Geometry check sheet. Reference: the model listing, model coordinates, mm. Face numbers are marked on the shaded views. Round coordinates to 2 decimals unless told otherwise and drop trailing zeros. Loops run counter-clockwise (first coordinate to the right, second up) from the corner with the lowest first, then second, coordinate; pieces in that order, holes last. Notation, with made-up numbers: (-33.5, 29) - (-13.5, 29) arc R16 ccw to (-13.5, 43) - close; hole circle Ø3 at (63.5, 43.25). An arc over 180 degrees is marked (long way). Answer as CSV lines item,"result". Start each with the question number.
1) Cross-section at C-C on x = -92.5. Record the boundary of the cut face in (y, z).
2) Cross-section at B-B on z = -218.5. Record the boundary of the cut face in (x, y).
3) Cross-section at A-A on y = 7. Record the boundary of the cut face in (x, z).
4) Draft check along X on the marked faces 1 and 2. Enter one of: released by +X, released by -X, zero draft, split by the parting line, or undercut.
5) Thickness scan on line 1 along X through (y, z) = (5.25, 234); line 2 along X through (y, z) = (9.25, -265); line 3 along Y through (x, z) = (-187.5, -121.5). Record the ranges inside material, lowest first.
6) Depth check by flat-ended pin: P1, Ø4.5, axis at x = -352, z = -127, coming from the -Y side; P2, Ø8, axis at x = -6, z = 194, coming from the +Y side. Enter the tip coordinate at first touch or a pass-through.
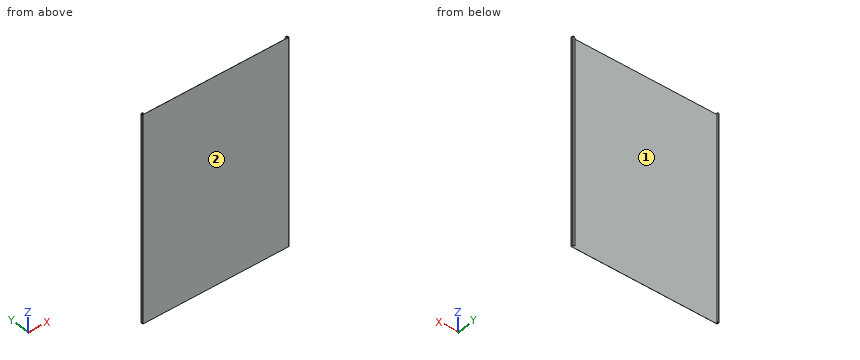
Autodesk Inventor part; units mm, degrees
ref_plane "YZ Plane" through (0, 0, 0) normal (1, 0, 0) x (0, 1, 0)
ref_plane "XZ Plane" through (0, 0, 0) normal (0, 1, 0) x (-1, 0, 0)
ref_plane "XY Plane" through (0, 0, 0) normal (0, 0, 1) x (1, 0, 0)
sketch "Sketch6" plane through (0, 0, 0) normal (0, 1, 0) x (-1, 0, 0)
  line L0 (356.7, -490) -> (-356.7, -490)
  line L1 (-356.7, -490) -> (-356.7, 490)
  line L2 (-356.7, 490) -> (356.7, 490)
  line L3 (356.7, 490) -> (356.7, -490)
  line L4 (356.7, -490) -> (-356.7, 490) construction
  line L5 (-356.7, -490) -> (356.7, 490) construction
  point P0 (0, 0)
  dimension "d52" = 713.4
  dimension "d53" = 980
extrude "Plate2" add sketch "Sketch6" along normal blind 0.5
sketch "Sketch11" plane through (-356.2, 0, 490) normal (-1, 0, 0) x (0, -1, 0)
  line L0 (0, -980) -> (0, 0)
  line L1 (0, 0) -> (-10, 0)
  line L2 (-10, 0) -> (-10, -980)
  line L3 (-10, -980) -> (0, -980)
edge flange "Flange2" height 10 angle 90 thickness 0.5 bend radius 0.5 thickness toward (-1, 0, 0) relief tear relief width 0.5 relief depth 0.25 edges at (-356.7, 0.5, 0) wall of the first edge with corners at (-356.2, 0, -490) (-356.2, 0, 490) (-356.2, 10, 490) (-356.2, 10, -490)
bend "Bend3"
corner "Corner3"
sketch "Sketch12" plane through (-356.7, 9.5, 490) normal (0, 1, 0) x (-1, 0, 0)
  line L0 (0, -980) -> (0, 0)
  line L1 (0, 0) -> (-10, 0)
  line L2 (-10, 0) -> (-10, -980)
  line L3 (-10, -980) -> (0, -980)
edge flange "Flange3" height 10 angle 90 thickness 0.5 bend radius 0.5 thickness toward (0, 1, 0) relief tear relief width 0.5 relief depth 0.25 edges at (-356.2, 10, 0) wall of the first edge with corners at (-356.7, 9.5, -490) (-356.7, 9.5, 490) (-346.7, 9.5, 490) (-346.7, 9.5, -490)
bend "Bend4"
corner "Corner4"
sketch "Sketch13" plane through (356.2, 0, -490) normal (1, 0, 0) x (0, 1, 0)
  line L0 (0, 980) -> (0, 0)
  line L1 (0, 0) -> (10, 0)
  line L2 (10, 0) -> (10, 980)
  line L3 (10, 980) -> (0, 980)
edge flange "Flange4" height 10 angle 90 thickness 0.5 bend radius 0.5 thickness toward (1, 0, 0) relief tear relief width 0.5 relief depth 0.25 edges at (356.7, 0.5, 0) wall of the first edge with corners at (356.2, 0, 490) (356.2, 0, -490) (356.2, 10, -490) (356.2, 10, 490)
bend "Bend5"
corner "Corner5"
sketch "Sketch14" plane through (356.7, 9.5, -490) normal (0, 1, 0) x (-1, 0, 0)
  line L0 (0, 980) -> (0, 0)
  line L1 (0, 0) -> (10, 0)
  line L2 (10, 0) -> (10, 980)
  line L3 (10, 980) -> (0, 980)
edge flange "Flange5" height 10 angle 90 thickness 0.5 bend radius 0.5 thickness toward (0, 1, 0) relief tear relief width 0.5 relief depth 0.25 edges at (356.2, 10, 0) wall of the first edge with corners at (356.7, 9.5, 490) (356.7, 9.5, -490) (346.7, 9.5, -490) (346.7, 9.5, 490)
bend "Bend6"
corner "Corner6"
fillet "Corner Round1" radius 4 4 edges at (346.7, 9.75, -490) (346.7, 9.75, 490) (-346.7, 9.75, -490) (-346.7, 9.75, 490)
equation "\"d52\" = ЖАБРЫ_базовая_ширина - 2 * ЖАБРЫ_шаг_листов"
equation "\"d53\" = ЖАБРЫ_базовая_длина_кор_лист"
equation "\"d54\" = Thickness"
equation "\"d84\" = BendReliefWidth"
equation "\"d85\" = BendReliefDepth"
equation "\"d86\" = MinimumRemnant"
equation "\"d87\" = TransitionRadius"
equation "\"d90\" = BendRadius"
equation "\"d91\" = CornerReliefSize"
equation "\"d92\" = GapSize"
equation "\"d93\" = JacobiRadiusSize"
equation "\"d94\" = BendReliefWidth"
equation "\"d95\" = BendReliefDepth"
equation "\"d96\" = MinimumRemnant"
equation "\"d97\" = TransitionRadius"
equation "\"d100\" = BendRadius"
equation "\"d101\" = CornerReliefSize"
equation "\"d102\" = GapSize"
equation "\"d103\" = JacobiRadiusSize"
equation "\"d104\" = BendReliefWidth"
equation "\"d105\" = BendReliefDepth"
equation "\"d106\" = MinimumRemnant"
equation "\"d107\" = TransitionRadius"
equation "\"d110\" = BendRadius"
equation "\"d111\" = CornerReliefSize"
equation "\"d112\" = GapSize"
equation "\"d113\" = JacobiRadiusSize"
equation "\"d114\" = BendReliefWidth"
equation "\"d115\" = BendReliefDepth"
equation "\"d116\" = MinimumRemnant"
equation "\"d117\" = TransitionRadius"
equation "\"d120\" = BendRadius"
equation "\"d121\" = CornerReliefSize"
equation "\"d122\" = GapSize"
equation "\"d123\" = JacobiRadiusSize"
equation "\"BendRadius\" = Thickness"
equation "\"BendReliefWidth\" = Thickness"
equation "\"BendReliefDepth\" = 0.5 * Thickness"
equation "\"CornerReliefSize\" = 4 * Thickness"
equation "\"MinimumRemnant\" = 2 * Thickness"
equation "\"TransitionRadius\" = BendRadius"
equation "\"JacobiRadiusSize\" = BendRadius"
equation "\"GapSize\" = Thickness"
properties part number "MSC 806 SHEET GILLS" material "Stainless Steel"
Answer block:
1,outline,"(0, -490) - (0.5, -490) - (0.5, 490) - (0, 490) - close"
2,outline,"(-356.7, 1) arc R1 ccw to (-355.7, 0) - (355.7, 0) arc R1 ccw to (356.7, 1) - (356.7, 9) arc R1 ccw to (355.7, 10) - (346.7, 10) - (346.7, 9.5) - (355.7, 9.5) arc R0.5 cw to (356.2, 9) - (356.2, 1) arc R0.5 cw to (355.7, 0.5) - (-355.7, 0.5) arc R0.5 cw to (-356.2, 1) - (-356.2, 9) arc R0.5 cw to (-355.7, 9.5) - (-346.7, 9.5) - (-346.7, 10) - (-355.7, 10) arc R1 ccw to (-356.7, 9) - close"
3,outline,"(-356.7, -490) - (-356.2, -490) - (-356.2, 490) - (-356.7, 490) - close; (356.2, -490) - (356.7, -490) - (356.7, 490) - (356.2, 490) - close"
4,face 1,"undercut"
4,face 2,"zero draft"
5,line 1,"x = -356.7 to -356.2, 356.2 to 356.7"
5,line 2,"x = -356.67 to -356.13, 356.13 to 356.67"
5,line 3,"y = 0 to 0.5"
6,P1,"stops at y = 0"
6,P2,"stops at y = 0.5"
